Source: CAD feature listing. Evaluate the final solid. Frame: model axes, mm. Give positions to 0.01 mm unless a question says otherwise; leave off trailing zeros. Write each loop counter-clockwise with the first axis right and the second up, starting at its lowest first coordinate (ties: lowest second). Pieces come first, ordered by that corner, then holes. Notation, with made-up numbers: M 44.5,80.5 L 79.5,80.5 A29 cw 79.5,117.5 Z; hole C -1,81 d3. An arc over 180 degrees is marked long. Return JSON: item names as keys, results as strings.
```python
from build123d import *

# Parameters (mm, degrees)
F0_R     = 5
F1_DEPTH = 2


with BuildPart() as f1:
    # F0 (on Top) → F1 (new body)
    with BuildSketch(Plane.XY):
        with BuildLine():
            Line((54.083269132, 10), (64.2261628933, 10))
            ThreePointArc((64.2261628933, 10), (0, 65), (-64.2261628933, 10))
            Line((-64.2261628933, 10), (-54.083269132, 10))
            ThreePointArc((-54.083269132, 10), (0, 55), (54.083269132, 10))
        make_face()
        with BuildLine():
            ThreePointArc((64.9830207232, -1.4856034775), (64.8720541596, 0), (64.9830207232, 1.4856034775))
            ThreePointArc((64.9830207232, 1.4856034775), (64.7447064998, 5.7552567496), (64.2261628933, 10))
            Line((64.2261628933, 10), (54.083269132, 10))
            ThreePointArc((54.083269132, 10), (54.7703377854, 5.0209659301), (55, 0))
            ThreePointArc((55, 0), (54.7703377854, -5.0209659301), (54.083269132, -10))
            Line((54.083269132, -10), (64.2261628933, -10))
            ThreePointArc((64.2261628933, -10), (64.7447064998, -5.7552567496), (64.9830207232, -1.4856034775))
        make_face()
        with BuildLine():
            ThreePointArc((64.2261628933, 10), (64.7447064998, 5.7552567496), (64.9830207232, 1.4856034775))
            ThreePointArc((64.9830207232, 1.4856034775), (68.3473332758, 7.5781275647), (74.8720541596, 10))
            Line((74.8720541596, 10), (64.2261628933, 10))
        make_face()
        with BuildLine():
            ThreePointArc((64.9830207232, 1.4856034775), (64.9957550422, 0.7428502521), (65, 0))
            ThreePointArc((65, 0), (64.9957550422, -0.7428502521), (64.9830207232, -1.4856034775))
            ThreePointArc((64.9830207232, -1.4856034775), (68.3473332758, -7.5781275647), (74.8720541596, -10))
            ThreePointArc((74.8720541596, -10), (81.9431219715, -7.0710678119), (84.8720541596, 0))
            ThreePointArc((84.8720541596, 0), (81.9431219715, 7.0710678119), (74.8720541596, 10))
            ThreePointArc((74.8720541596, 10), (68.3473332758, 7.5781275647), (64.9830207232, 1.4856034775))
        make_face()
        with Locations((74.8720541596, 0)):
            Circle(F0_R, mode=Mode.SUBTRACT)
        with BuildLine():
            ThreePointArc((74.8720541596, -10), (68.3473332758, -7.5781275647), (64.9830207232, -1.4856034775))
            ThreePointArc((64.9830207232, -1.4856034775), (64.7447064998, -5.7552567496), (64.2261628933, -10))
            Line((64.2261628933, -10), (74.8720541596, -10))
        make_face()
        with BuildLine():
            ThreePointArc((-64.2261628933, -10), (0, -65), (64.2261628933, -10))
            Line((64.2261628933, -10), (54.083269132, -10))
            ThreePointArc((54.083269132, -10), (0, -55), (-54.083269132, -10))
            Line((-54.083269132, -10), (-64.2261628933, -10))
        make_face()
        with BuildLine():
            ThreePointArc((-64.9992465548, -0.3129653476), (-65, 0), (-64.9992465548, 0.3129653476))
            ThreePointArc((-64.9992465548, 0.3129653476), (-68.0348097105, 7.1808653338), (-74.9943480303, 10))
            ThreePointArc((-74.9943480303, 10), (-84.9943479896, -1.92e-08), (-74.994347992, -10))
            ThreePointArc((-74.994347992, -10), (-68.0348096967, -7.1808653204), (-64.9992465548, -0.3129653476))
        make_face()
        with Locations((-74.9943479896, 0)):
            Circle(F0_R, mode=Mode.SUBTRACT)
        with BuildLine():
            Line((-74.994347992, -10), (-64.2261628933, -10))
            ThreePointArc((-64.2261628933, -10), (-64.7939910165, -5.1709504109), (-64.9992465548, -0.3129653476))
            ThreePointArc((-64.9992465548, -0.3129653476), (-68.0348096967, -7.1808653204), (-74.994347992, -10))
        make_face()
        with BuildLine():
            ThreePointArc((-64.9992465548, 0.3129653476), (-64.7939910165, 5.1709504109), (-64.2261628933, 10))
            Line((-64.2261628933, 10), (-74.9943480303, 10))
            ThreePointArc((-74.9943480303, 10), (-68.0348097105, 7.1808653338), (-64.9992465548, 0.3129653476))
        make_face()
        with BuildLine():
            Line((-54.083269132, 10), (-64.2261628933, 10))
            ThreePointArc((-64.2261628933, 10), (-64.7939910165, 5.1709504109), (-64.9992465548, 0.3129653476))
            ThreePointArc((-64.9992465548, 0.3129653476), (-64.9955727059, 0.1565018408), (-64.9943479896, 0))
            ThreePointArc((-64.9943479896, 0), (-64.9955727059, -0.1565018408), (-64.9992465548, -0.3129653476))
            ThreePointArc((-64.9992465548, -0.3129653476), (-64.7939910165, -5.1709504109), (-64.2261628933, -10))
            Line((-64.2261628933, -10), (-54.083269132, -10))
            ThreePointArc((-54.083269132, -10), (-55, 0), (-54.083269132, 10))
        make_face()
        with BuildLine():
            ThreePointArc((-64.9943479896, 0), (-64.9955727059, 0.1565018408), (-64.9992465548, 0.3129653476))
            ThreePointArc((-64.9992465548, 0.3129653476), (-65, 0), (-64.9992465548, -0.3129653476))
            ThreePointArc((-64.9992465548, -0.3129653476), (-64.9955727059, -0.1565018408), (-64.9943479896, 0))
        make_face()
        with BuildLine():
            ThreePointArc((64.9830207232, -1.4856034775), (64.9957550422, -0.7428502521), (65, 0))
            ThreePointArc((65, 0), (64.9957550422, 0.7428502521), (64.9830207232, 1.4856034775))
            ThreePointArc((64.9830207232, 1.4856034775), (64.8720541596, 0), (64.9830207232, -1.4856034775))
        make_face()
    extrude(amount=F1_DEPTH)


solid = f1.part
```
1) Cut plane B-B, the plane z = 1.5. Return the cut outline in (x, y), then the cut area to 3 significant figures.
Numbers:
{"outline": "M -74.99,-10 L -64.23,-10 A65 ccw 64.23,-10 L 74.87,-10 A10 ccw 74.87,10 L 64.23,10 A65 ccw -64.23,10 L -74.99,10 A10 ccw Z; hole C -74.99,0 d10; hole C 0,0 d110; hole C 74.87,0 d10", "area": "4,330 mm²"}
2) Cut plane D-D, the plane x = -58.5. Return the cut outline in (y, z).
Numbers:
{"outline": "M -28.33,0 L 28.33,0 L 28.33,2 L -28.33,2 Z"}
3) Cut plane C-C, the plane x = 22. Return the cut outline in (y, z), then the cut area to 3 significant figures.
Numbers:
{"outline": "M -61.16,0 L -50.41,0 L -50.41,2 L -61.16,2 Z; M 50.41,0 L 61.16,0 L 61.16,2 L 50.41,2 Z", "area": "43.0 mm²"}
4) Contact query for flat-ended pins moving along their axis: pin 1 Ø0.6 at (x, z) = (-71, 1) entering from +Y; pin 2 Ø1 at (x, z) = (-40, 0.5) entering from -Y; pin 3 Ø1 at (x, z) = (-68, 1) entering from -Y. Output: stop coordinate, or through.
Numbers:
{"pin 1": "stops at y = 10", "pin 2": "stops at y = -51.62", "pin 3": "stops at y = -10"}
5) Draft query along Y for faces 1 (the face through (79.49, -1.92, 0.99)), 2 (the face through (1.289, 64.987, 0.986)), 3 (the face through (-84.99, 0.22, 0.99)). Return one class per face: released by +Y, released by -Y, zero draft, split by the parting line, or undercut.
Numbers:
{"face 1": "undercut", "face 2": "released by +Y", "face 3": "split by the parting line"}
6) Cut plane A-A, the plane y = 33. Return the cut outline in (x, z).
Numbers:
{"outline": "M -56,0 L -44,0 L -44,2 L -56,2 Z; M 44,0 L 56,0 L 56,2 L 44,2 Z"}
7) Line query: line 1 (Y direction, x = -75, z = 0.5); line 2 (X direction, y = 34, z = 1.3); line 3 (X direction, y = 1, z = 0.95). Output: solid intervals per line, ascending. Write a range as [from, to].
Numbers:
{"line 1": "y = [-10, -5], [5, 10]", "line 2": "x = [-55.4, -43.23], [43.23, 55.4]", "line 3": "x = [-84.94, -79.89], [-70.1, -54.99], [54.99, 69.97], [79.77, 84.82]"}
